CAD build for the part. Positions are in the model's coordinates, mm. Face numbers are marked on the shaded views. A direction names the side the tool comes from. Round coordinates to 2 decimals unless told otherwise and drop trailing zeros. Loops run counter-clockwise (first coordinate to the right, second up) from the corner with the lowest first, then second, coordinate; pieces in that order, holes last. Notation, with made-up numbers: (-20.75, 39.5) -> (-11.75, 39.5) arc R13 cw to (-11.75, 60.5) -> close; hole circle Ø10 at (26, 87). An arc over 180 degrees is marked (long way). Answer as CSV lines item,"result".
```python
from build123d import *

# Parameters (mm, degrees)
KREUZSCHLITZ1_H_DEPTH      = 0.4
KREUZSCHLITZ1_H_DEPTH_BACK = 0.4
KREUZSCHLITZ2_H_DEPTH      = 0.4
KREUZSCHLITZ2_H_DEPTH_BACK = 0.4
BOSS_EXTRUDE1_START        = 2
SKETCH1_R                  = 1.1935
BOSS_EXTRUDE1_DEPTH        = 2
CUT_EXTRUDE1_DEPTH         = 2
CUT_EXTRUDE1_DEPTH_BACK    = 2
SKETCH2_W                  = 2.387
SKETCH2_H                  = 5


with BuildPart() as part:
    # Skizze1 → Basis-Rotation (revolve)
    with BuildSketch(Plane.XY, mode=Mode.PRIVATE) as basis_rotation_sk:
        Polygon((0, 0), (2.75, 0), (2.75, -0.2375), (1.5, -1.4875), (1.5, -1.9875), (1.3375, -1.9875), (1.3375, -2.112584684), (1.1935, -2.65), (1.1935, -8), (0, -8), align=None)
    revolve(basis_rotation_sk.sketch.rotate(Axis((0, 0, 0), (0, -1, 0)), 180), axis=Axis((0, 0, 0), (0, -1, 0)))

    # Skizze2 → Kreuzschlitz1 H (cut, two sides: drawn at the far end of the back side and taken through both)
    with BuildSketch(Plane.XY.offset(-KREUZSCHLITZ1_H_DEPTH_BACK)):
        Polygon((-0.55, -2.1), (0.55, -2.1), (1.6, -1.05), (1.6, 0), (-1.6, 0), (-1.6, -1.05), align=None)
    extrude(amount=KREUZSCHLITZ1_H_DEPTH + KREUZSCHLITZ1_H_DEPTH_BACK, mode=Mode.SUBTRACT)

    # Skizze3 → Kreuzschlitz2 H (cut, two sides: drawn at the far end of the back side and taken through both)
    with BuildSketch(Plane(origin=(0, 0, 0), x_dir=(0, 0, -1), z_dir=(1, 0, 0)).offset(-KREUZSCHLITZ2_H_DEPTH_BACK)):
        Polygon((-0.55, -2.1), (0.55, -2.1), (1.6, -1.05), (1.6, 0), (-1.6, 0), (-1.6, -1.05), align=None)
    extrude(amount=KREUZSCHLITZ2_H_DEPTH + KREUZSCHLITZ2_H_DEPTH_BACK, mode=Mode.SUBTRACT)

    # Sketch1 → Boss-Extrude1 (add)
    with BuildSketch(Plane.XZ.offset(8).offset(BOSS_EXTRUDE1_START)):
        with Locations(Location((0, 0, 0), (0, 0, 180))):
            Circle(SKETCH1_R)
    extrude(amount=-BOSS_EXTRUDE1_DEPTH)

    # Sketch2 → Cut-Extrude1 (cut, two sides: drawn at the far end of the back side and taken through both)
    with BuildSketch(Plane(origin=(0, 0, 0), x_dir=(0, 0, -1), z_dir=(1, 0, 0)).offset(-CUT_EXTRUDE1_DEPTH_BACK)):
        with Locations((0, -7.5)):
            Rectangle(SKETCH2_W, SKETCH2_H)
    extrude(amount=CUT_EXTRUDE1_DEPTH + CUT_EXTRUDE1_DEPTH_BACK, mode=Mode.SUBTRACT)


solid = part.part
```
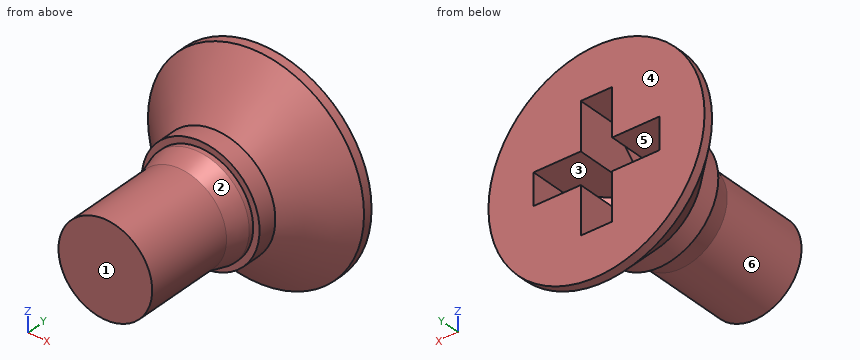
Q1. Slice it at B-B, the plane y = -1.35. Give the cut face in (x, z) (1 decimal), and give its area (3 significant figures).
Results:
outline,"circle Ø3.3 at (0, 0); hole (-1.3, -0.4) -> (-0.4, -0.4) -> (-0.4, -1.3) -> (0.4, -1.3) -> (0.4, -0.4) -> (1.3, -0.4) -> (1.3, 0.4) -> (0.4, 0.4) -> (0.4, 1.3) -> (-0.4, 1.3) -> (-0.4, 0.4) -> (-1.3, 0.4) -> close"
area,"4.90 mm2"
Q2. Two-plate mould, pull along X, no slides. Class the marked faces 1, 2 and 3: pulls with the +X half, pulls with the -X half, needs draft (parallel to the pull), parting line crosses it, or undercut.
Results:
face 1,"needs draft"
face 2,"parting line crosses it"
face 3,"undercut"
Q3. Drop flat-ended pins along their axis: pin 1 Ø1.5 at (y, z) = (-1.5, 0) entering from -X; pin 2 Ø0.6 at (x, y) = (1, -1) entering from +Z; pin 3 Ø1 at (y, z) = (-1, 1) entering from +X. Give the stop position or say it passes through.
Results:
pin 1,"x = -2.24"
pin 2,"z = 2.08"
pin 3,"x = 2.31"
Q4. Slice it at D-D, the plane y = -4.3. Give the cut face in (x, z).
Results:
outline,"circle Ø2.39 at (0, 0)"
Q5. Tool access for the marked faces 4, 5 and 6: list every direction of +Z, -Z, +X, -X, +Y, -Y with a clear straight run to the whole face (end or side of a thin tool).
Results:
face 4,"+Z, -Z, +X, -X, +Y"
face 5,"+Y"
face 6,"-Y"
Q6. Slice it at C-C, the plane x = 0. Give the cut face in (y, z), and give its area (3 significant figures).
Results:
outline,"(-5, -1.19) -> (-2.65, -1.19) -> (-2.11, -1.34) -> (-1.99, -1.34) -> (-1.99, -1.5) -> (-1.49, -1.5) -> (-0.24, -2.75) -> (0, -2.75) -> (0, -1.6) -> (-1.05, -1.6) -> (-2.1, -0.55) -> (-2.1, 0.55) -> (-1.05, 1.6) -> (0, 1.6) -> (0, 2.75) -> (-0.24, 2.75) -> (-1.49, 1.5) -> (-1.99, 1.5) -> (-1.99, 1.34) -> (-2.11, 1.34) -> (-2.65, 1.19) -> (-5, 1.19) -> close"
area,"9.81 mm2"
Q7. Slice it at A-A, the plane z = 0. Give the cut face in (x, y), and give its area (3 significant figures).
Results:
outline,"(-2.75, -0.24) -> (-1.5, -1.49) -> (-1.5, -1.99) -> (-1.34, -1.99) -> (-1.34, -2.11) -> (-1.19, -2.65) -> (-1.19, -5) -> (1.19, -5) -> (1.19, -2.65) -> (1.34, -2.11) -> (1.34, -1.99) -> (1.5, -1.99) -> (1.5, -1.49) -> (2.75, -0.24) -> (2.75, 0) -> (1.6, 0) -> (1.6, -1.05) -> (0.55, -2.1) -> (-0.55, -2.1) -> (-1.6, -1.05) -> (-1.6, 0) -> (-2.75, 0) -> close"
area,"9.81 mm2"
Q8. Probe L1, parallel to Y at x = -2.15, z = 1.15; L2, parallel to Y at x = 0.1, z = -0.05; L3, parallel to X at y = -0.6, z = 1. List the from-to ranges inside material, lowest first. Write a range as [from, to].
Results:
L1,"[-0.55, 0]"
L2,"[-5, -2.1]"
L3,"[-2.17, -0.4], [0.4, 2.17]"
